Check sheet for the modelled part. Datum: model origin and axes. Units: mm. Face numbers are marked on the shaded views. A direction names the side the tool comes from. Coordinates: 2 decimals unless noted, no trailing zeros. Loops run counter-clockwise (first coordinate to the right, second up) from the corner with the lowest first, then second, coordinate; pieces in that order, holes last. Notation, with made-up numbers: M 83,41 L 95,41 A21 ccw 95,54 Z; hole C -34,62 d3. An arc over 180 degrees is marked long. Write each question's results on one line, items separated by ' | '. Start each with the question number.
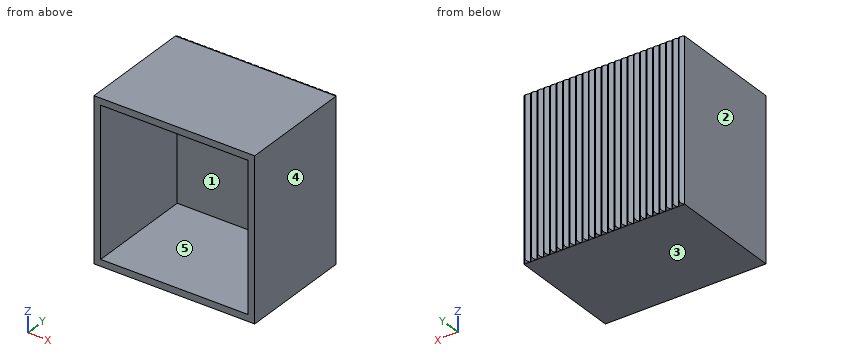
from build123d import *

# Parameters (mm, degrees)
SKETCH1_W           = 60
SKETCH1_H           = 60
SKETCH1_W_2         = 55
SKETCH1_H_2         = 55
BOSS_EXTRUDE1_DEPTH = 40
SKETCH2_W           = 60
SKETCH2_H           = 60
BOSS_EXTRUDE2_DEPTH = 2.5
BOSS_EXTRUDE3_DEPTH = 60
CUT_EXTRUDE1_REACH  = 82.061


with BuildPart() as part:
    # Sketch1 → Boss-Extrude1 (new body)
    with BuildSketch(Plane(origin=(0, 0, 0), x_dir=(1, 0, 0), z_dir=(0, 1, 0))):
        Rectangle(SKETCH1_W, SKETCH1_H)
        Rectangle(SKETCH1_W_2, SKETCH1_H_2, mode=Mode.SUBTRACT)
    extrude(amount=BOSS_EXTRUDE1_DEPTH)

    # Sketch2 → Boss-Extrude2 (add)
    with BuildSketch(Plane(origin=(0, 40, 0), x_dir=(1, 0, 0), z_dir=(0, 1, 0))):
        Rectangle(SKETCH2_W, SKETCH2_H)
    extrude(amount=BOSS_EXTRUDE2_DEPTH)

    # Sketch3 → Boss-Extrude3 (add)
    with BuildSketch(Plane(origin=(0, 0, -30), x_dir=(-1, 0, 0), z_dir=(0, 0, -1))):
        Polygon((-30, 42.5), (-28.8, 43.7), (-27.6, 42.5), (-26.4, 43.7), (-25.2, 42.5), (-24, 43.7), (-22.8, 42.5), (-21.6, 43.7), (-20.4, 42.5), (-19.2, 43.7), (-18, 42.5), (-16.8, 43.7), (-15.6, 42.5), (-14.4, 43.7), (-13.2, 42.5), (-12, 43.7), (-10.8, 42.5), (-9.6, 43.7), (-8.4, 42.5), (-7.2, 43.7), (-6, 42.5), (-4.8, 43.7), (-3.6, 42.5), (-2.4, 43.7), (-1.2, 42.5), (0, 43.7), (1.2, 42.5), (2.4, 43.7), (3.6, 42.5), (4.8, 43.7), (6, 42.5), (7.2, 43.7), (8.4, 42.5), (9.6, 43.7), (10.8, 42.5), (12, 43.7), (13.2, 42.5), (14.4, 43.7), (15.6, 42.5), (16.8, 43.7), (18, 42.5), (19.2, 43.7), (20.4, 42.5), (21.6, 43.7), (22.8, 42.5), (24, 43.7), (25.2, 42.5), (26.4, 43.7), (27.6, 42.5), (28.8, 43.7), (30, 42.5), (30, 42.170064374), (-30, 42.170064374), align=None)
    extrude(amount=-BOSS_EXTRUDE3_DEPTH)

    # Cut-Extrude1: up to this face of the body (flat: up to its plane)
    cut_extrude1_end = Plane(part.part.faces().sort_by_distance((30, 21.25, 0))[0])
    # Sketch4 → Cut-Extrude1 (cut, up to the picked face)
    with BuildSketch(Plane.ZY.offset(30), mode=Mode.PRIVATE) as cut_extrude1_sk1:
        with BuildLine():
            Line((-30, 42.5), (-30, 43.7))
            Line((-30, 43.7), (-28.8, 43.7))
            ThreePointArc((-28.8, 43.7), (-29.648528137, 43.348528137), (-30, 42.5))
        make_face()
    cut_extrude1_tool1 = split(extrude(cut_extrude1_sk1.sketch, amount=-CUT_EXTRUDE1_REACH, mode=Mode.PRIVATE), bisect_by=cut_extrude1_end, keep=Keep.BOTH, mode=Mode.PRIVATE)
    cut_extrude1 = cut_extrude1_tool1.solids().sort_by(Axis((-30, 43.431958, -29.731958), (1, 0, 0)))[0]
    add(cut_extrude1, mode=Mode.SUBTRACT)

    # Mirror1: Cut-Extrude1 across plane
    add(cut_extrude1.mirror(Plane.XY), mode=Mode.SUBTRACT)


solid = part.part
1) Set-up check for the marked faces 1 and 2: record each of +Z, -Z, +X, -X, +Y, -Y from which the full face is reachable in a straight line by a thin tool's end or side.
2) Thickness scan on probe 1 along Z at (x, y) = (-4, 9); probe 2 along Y at (x, z) = (0.5, 11). Record the ranges inside material, lowest first.
3) Gauge pin test, flat end, axial feed: P1, Ø1, axis at x = -23.5, z = -11, coming from the -Y side. Record the tip position at first contact, or that the pin passes through.
4) Section check A-A (y = 23.5). Enter the section's corners in (x, z), then the cut area to 3 significant figures.
5) Release check for a two-part mould opening along Z. For the marked faces 3, 4 and 5 record: +Z half, -Z half, draft (parallel to the pull), parting line (faces both ways), or undercut.
Return value:
1) face 1: -Y | face 2: +Z, -Z, -X, +Y, -Y
2) probe 1: z = -30 to -27.5, 27.5 to 30 | probe 2: y = 40 to 43.2
3) P1: stops at y = 40
4) outline: M -30,-30 L 30,-30 L 30,30 L -30,30 Z; hole M -27.5,-27.5 L 27.5,-27.5 L 27.5,27.5 L -27.5,27.5 Z | area: 575 mm2
5) face 3: -Z half | face 4: draft | face 5: undercut
